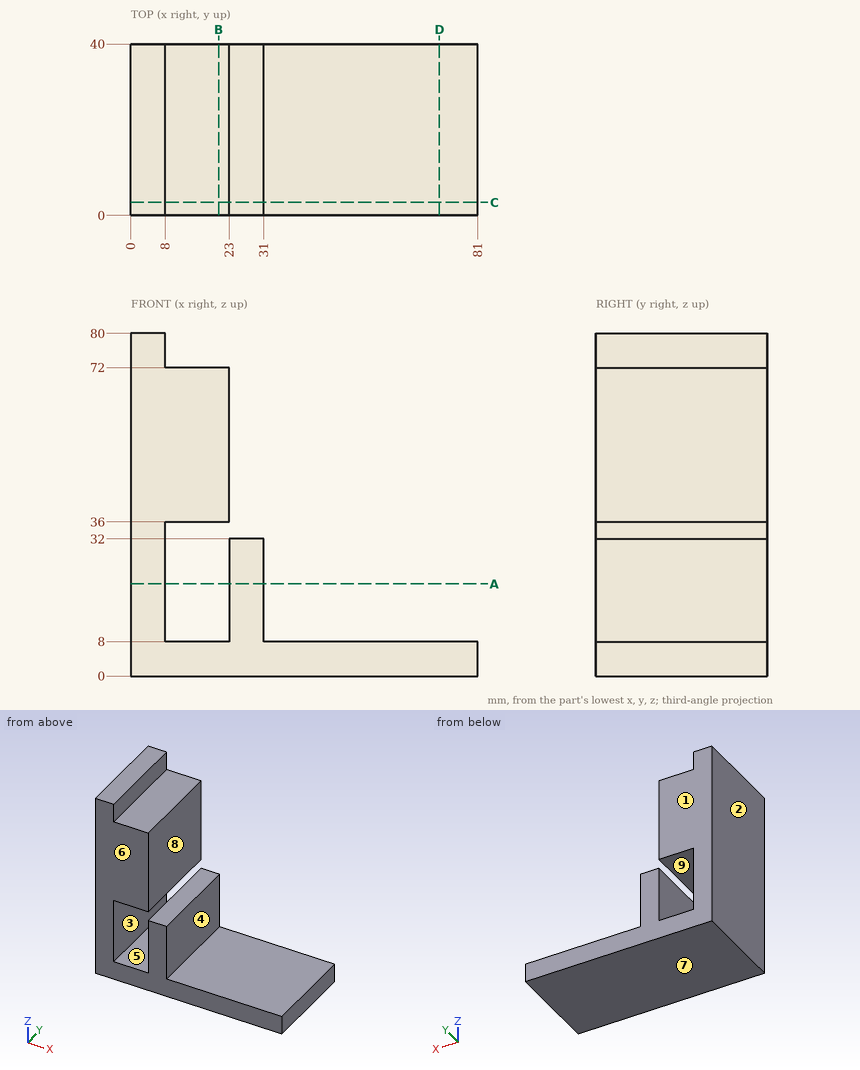
Geometry: see drawing. Coordinates: mm, zero at the bounding-box minimum. A direction names the side the tool comes from. Round coordinates to 2 decimals unless told otherwise and drop trailing zeros. Write each loop counter-clockwise with the first axis right and the second up, starting at its lowest first coordinate (ties: lowest second). Pieces come first, ordered by that corner, then holes.
1) Cut plane B-B (x = 20.5). Return the cut outline in (y, z), then the cut area to 3 significant figures.
2) Reachability of the marked faces 5, 6, 7, 8 and 9 from +Z, -Z, +X, -X, +Y, -Y: full face, straight path, thin tool, end or side. Return the list, or none.
3) Draft query along X for the marked faces 1, 2, 3 and 4. Return one class per face: pulls with the +X half, pulls with the -X half, needs draft (parallel to the pull), parting line crosses it, or undercut.
4) Cut plane D-D (x = 72). Return the cut outline in (y, z).
5) Ray query, L1, parallel to X at y = 6, z = 22; L2, parallel to Z at x = 9, y = 15.5; L3, parallel to X at y = 2, z = 38.5. Return the intervals inside material, ascending.
6) Cut plane C-C (y = 3). Return the cut outline in (x, z), then the cut area to 3 significant figures.
7) Contact query for flat-ended pins moving along their axis: P1, Ø9, axis at x = 26.5, y = 23.5, coming from the +Z side; P2, Ø22.5, axis at y = 26, z = 20.5, coming from the +X side; P3, Ø10, axis at x = 61.5, y = 26, coming from the +Z side. Output: stop coordinate, or through.
8) Cut plane A-A (z = 21.5). Return the cut outline in (x, y).
Geometry says:
1. outline: (0, 0) - (40, 0) - (40, 8) - (0, 8) - close; (0, 36) - (40, 36) - (40, 72) - (0, 72) - close
1. area: 1,760 mm2
2. face 5: +Y, -Y
2. face 6: +Z, -Z, +X, -X, -Y
2. face 7: -Z, +X, -X, +Y, -Y
2. face 8: +Z, +X, +Y, -Y
2. face 9: +X, +Y, -Y
3. face 1: needs draft
3. face 2: pulls with the -X half
3. face 3: undercut
3. face 4: pulls with the +X half
4. outline: (0, 0) - (40, 0) - (40, 8) - (0, 8) - close
5. L1: x = 0 to 8, 23 to 31
5. L2: z = 0 to 8, 36 to 72
5. L3: x = 0 to 23
6. outline: (0, 0) - (81, 0) - (81, 8) - (31, 8) - (31, 32) - (23, 32) - (23, 8) - (8, 8) - (8, 36) - (23, 36) - (23, 72) - (8, 72) - (8, 80) - (0, 80) - close
6. area: 1,960 mm2
7. P1: stops at z = 72
7. P2: stops at x = 31
7. P3: stops at z = 8
8. outline: (0, 0) - (8, 0) - (8, 40) - (0, 40) - close; (23, 0) - (31, 0) - (31, 40) - (23, 40) - close
